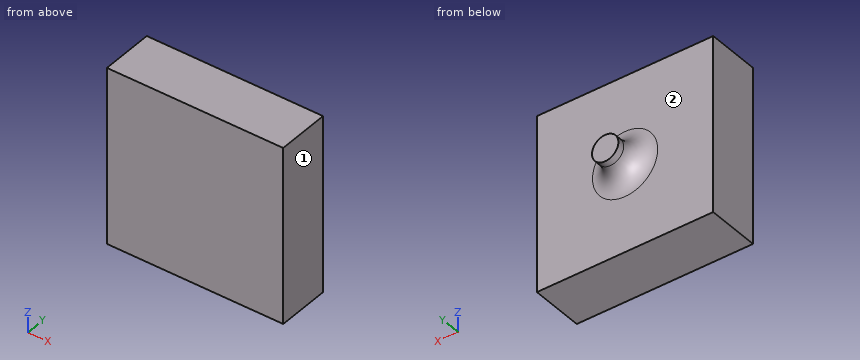
from build123d import *

# Parameters (mm, degrees)
SKETCH_1_W      = 10
SKETCH_1_H      = 10
EXTRUDE_1_DEPTH = 3
SKETCH_2_R      = 0.75
EXTRUDE_2_DEPTH = 1.5
FILLET_1_R      = 1.1


with BuildPart() as part:
    # 草图1 → 凸台-拉伸1 (new body)
    with BuildSketch(Plane(origin=(0, 0, 0), x_dir=(1, 0, 0), z_dir=(0, 1, 0))):
        Rectangle(SKETCH_1_W, SKETCH_1_H)
    extrude(amount=EXTRUDE_1_DEPTH)

    # 草图2 → 凸台-拉伸2 (add)
    with BuildSketch(Plane(origin=(0, 3, 0), x_dir=(1, 0, 0), z_dir=(0, 1, 0))):
        Circle(SKETCH_2_R)
    extrude(amount=EXTRUDE_2_DEPTH)

    # 圆角1
    fillet_1_edges = [part.edges().sort_by_distance(p)[0] for p in [
        (-0.75, 3, 0),
    ]]
    fillet(fillet_1_edges, radius=FILLET_1_R)


solid = part.part
Input: part model. Units: mm. Frame: model coordinates. Face numbers are marked on the shaded views. A direction names the side the tool comes from. Round coordinates to 2 decimals unless told otherwise and drop trailing zeros. Write each loop counter-clockwise with the first axis right and the second up, starting at its lowest first coordinate (ties: lowest second). Pieces come first, ordered by that corner, then holes.
1) Cut plane C-C (y = 3.8). Return the cut outline in (x, z).
2) Cut plane B-B (z = 0). Return the cut outline in (x, y).
3) Reachability of the marked faces 1 and 2 from +Z, -Z, +X, -X, +Y, -Y: full face, straight path, thin tool, end or side. Return the list, or none.
4) Ray query, L1, parallel to Y at x = 2.75, z = 2; L2, parallel to Y at x = 1.5, z = 0.25; L3, parallel to Z at x = -0.5, y = 4.3. Return the intervals inside material, ascending.
5) Cut plane A-A (x = 0). Return the cut outline in (y, z).
6) Contact query for a flat-ended pin moving along its axis: P1, Ø5, axis at x = 3, z = 3, coming from the +Y side. Output: stop coordinate, or through.
7) Cut plane D-D (x = 3.5). Return the cut outline in (y, z).
Geometry says:
1. outline: circle Ø1.58 at (0, 0)
2. outline: (-5, 0) - (5, 0) - (5, 3) - (1.85, 3) arc R1.1 cw to (0.75, 4.1) - (0.75, 4.5) - (-0.75, 4.5) - (-0.75, 4.1) arc R1.1 cw to (-1.85, 3) - (-5, 3) - close
3. face 1: +Z, -Z, +X, +Y, -Y
3. face 2: +Y
4. L1: y = 0 to 3
4. L2: y = 0 to 3.05
4. L3: z = -0.56 to 0.56
5. outline: (0, -5) - (3, -5) - (3, -1.85) arc R1.1 cw to (4.1, -0.75) - (4.5, -0.75) - (4.5, 0.75) - (4.1, 0.75) arc R1.1 cw to (3, 1.85) - (3, 5) - (0, 5) - close
6. P1: stops at y = 3.01
7. outline: (0, -5) - (3, -5) - (3, 5) - (0, 5) - close
